The listing builds one solid part. Answer for the finished solid, in the listing's coordinates (mm). A direction names the side the tool comes from. Coordinates: 2 decimals unless noted, no trailing zeros. Write each loop counter-clockwise with the first axis right and the second up, starting at its lowest first coordinate (ties: lowest second). Pieces come first, ordered by that corner, then holes. Notation, with made-up numbers: M 55,40 L 89,40 A6 cw 89,47 Z; hole C 7,51.5 d2. An arc over 180 degrees is marked long. Answer as CSV lines item,"result".
```python
from build123d import *

# Parameters (mm, degrees)
SKETCH1_W           = 54.8
SKETCH1_H           = 53.53
BOSS_EXTRUDE1_DEPTH = 41.6
SKETCH2_W           = 51.6
SKETCH2_H           = 50.33
CUT_EXTRUDE1_DEPTH  = 39.6
SKETCH3_W           = 5.48
SKETCH3_H           = 5.48
BOSS_EXTRUDE2_DEPTH = 25
SKETCH4_R           = 1.35
CUT_EXTRUDE2_DEPTH  = 10
CUT_EXTRUDE3_REACH  = 43.6
SKETCH5_R           = 3.5
CUT_EXTRUDE4_REACH  = 43.6
SKETCH6_R           = 3.1
CUT_EXTRUDE5_REACH  = 43.6
SKETCH7_R           = 3.6
CUT_EXTRUDE6_REACH  = 56.8
SKETCH8_R           = 1.25
CUT_EXTRUDE7_REACH  = 56.8
SKETCH10_R          = 1.25
CUT_EXTRUDE8_REACH  = 55.53
SKETCH12_R          = 7.680495542
CUT_EXTRUDE9_REACH  = 55.53
SKETCH13_W          = 22.581735489
SKETCH13_H          = 15.862362247
CUT_EXTRUDE10_REACH = 56.8
SKETCH14_R          = 1.25


with BuildPart() as part:
    # Sketch1 → Boss-Extrude1 (new body)
    with BuildSketch(Plane(origin=(0, 0, 0), x_dir=(1, 0, 0), z_dir=(0, 1, 0))):
        Rectangle(SKETCH1_W, SKETCH1_H)
    extrude(amount=BOSS_EXTRUDE1_DEPTH)

    # Sketch2 → Cut-Extrude1 (cut)
    with BuildSketch(Plane(origin=(0, 41.6, 0), x_dir=(1, 0, 0), z_dir=(0, 1, 0))):
        Rectangle(SKETCH2_W, SKETCH2_H)
    extrude(amount=-CUT_EXTRUDE1_DEPTH, mode=Mode.SUBTRACT)

    # Sketch3 → Boss-Extrude2 (add)
    with BuildSketch(Plane(origin=(0, 2, 0), x_dir=(1, 0, 0), z_dir=(0, 1, 0))):
        with Locations((-23.06, 22.425)):
            Rectangle(SKETCH3_W, SKETCH3_H)
        with Locations((23.06, 22.425)):
            Rectangle(SKETCH3_W, SKETCH3_H)
        with Locations((23.06, -22.425)):
            Rectangle(SKETCH3_W, SKETCH3_H)
    extrude(amount=BOSS_EXTRUDE2_DEPTH)

    # Sketch4 → Cut-Extrude2 (cut)
    with BuildSketch(Plane(origin=(0, 27, 0), x_dir=(1, 0, 0), z_dir=(0, 1, 0))):
        with Locations((-22.86, 22.225)):
            Circle(SKETCH4_R)
        with Locations((22.86, 22.225)):
            Circle(SKETCH4_R)
        with Locations((22.86, -22.217113742)):
            Circle(SKETCH4_R)
    extrude(amount=-CUT_EXTRUDE2_DEPTH, mode=Mode.SUBTRACT)

    # Sketch5 → Cut-Extrude3 (cut, up to next)
    with BuildSketch(Plane(origin=(0, 0, 0), x_dir=(-1, 0, 0), z_dir=(0, -1, 0)), mode=Mode.PRIVATE) as cut_extrude3_sk1:
        with Locations((-12.762863618, 17.186859774)):
            Circle(SKETCH5_R)
    cut_extrude3_tool1 = extrude(cut_extrude3_sk1.sketch, amount=-CUT_EXTRUDE3_REACH, mode=Mode.PRIVATE) & part.part
    add(cut_extrude3_tool1.solids().sort_by_distance((12.762864, 0, -17.18686))[0], mode=Mode.SUBTRACT)
    # Sketch5 → Cut-Extrude3 (cut, up to next)
    with BuildSketch(Plane(origin=(0, 0, 0), x_dir=(-1, 0, 0), z_dir=(0, -1, 0)), mode=Mode.PRIVATE) as cut_extrude3_sk2:
        with Locations((12.108357792, 17.186859774)):
            Circle(SKETCH5_R)
    cut_extrude3_tool2 = extrude(cut_extrude3_sk2.sketch, amount=-CUT_EXTRUDE3_REACH, mode=Mode.PRIVATE) & part.part
    add(cut_extrude3_tool2.solids().sort_by_distance((-12.108358, 0, -17.18686))[0], mode=Mode.SUBTRACT)

    # Sketch6 → Cut-Extrude4 (cut, up to next)
    with BuildSketch(Plane(origin=(0, 0, 0), x_dir=(-1, 0, 0), z_dir=(0, -1, 0)), mode=Mode.PRIVATE) as cut_extrude4_sk1:
        with Locations((-16.908067186, 1.527180262)):
            Circle(SKETCH6_R)
    cut_extrude4_tool1 = extrude(cut_extrude4_sk1.sketch, amount=-CUT_EXTRUDE4_REACH, mode=Mode.PRIVATE) & part.part
    add(cut_extrude4_tool1.solids().sort_by_distance((16.908067, 0, -1.52718))[0], mode=Mode.SUBTRACT)
    # Sketch6 → Cut-Extrude4 (cut, up to next)
    with BuildSketch(Plane(origin=(0, 0, 0), x_dir=(-1, 0, 0), z_dir=(0, -1, 0)), mode=Mode.PRIVATE) as cut_extrude4_sk2:
        with Locations((-8.726744354, 1.527180262)):
            Circle(SKETCH6_R)
    cut_extrude4_tool2 = extrude(cut_extrude4_sk2.sketch, amount=-CUT_EXTRUDE4_REACH, mode=Mode.PRIVATE) & part.part
    add(cut_extrude4_tool2.solids().sort_by_distance((8.726744, 0, -1.52718))[0], mode=Mode.SUBTRACT)

    # Sketch7 → Cut-Extrude5 (cut, up to next)
    with BuildSketch(Plane(origin=(0, 0, 0), x_dir=(-1, 0, 0), z_dir=(0, -1, 0)), mode=Mode.PRIVATE) as cut_extrude5_sk1:
        with Locations((-12.653779314, -10.035756007)):
            Circle(SKETCH7_R)
    cut_extrude5_tool1 = extrude(cut_extrude5_sk1.sketch, amount=-CUT_EXTRUDE5_REACH, mode=Mode.PRIVATE) & part.part
    add(cut_extrude5_tool1.solids().sort_by_distance((12.653779, 0, 10.035756))[0], mode=Mode.SUBTRACT)

    # Sketch8 → Cut-Extrude6 (cut, up to next)
    with BuildSketch(Plane(origin=(27.4, 0, 0), x_dir=(0, 0, -1), z_dir=(1, 0, 0)), mode=Mode.PRIVATE) as cut_extrude6_sk1:
        with Locations((-21.585, 36.49)):
            Circle(SKETCH8_R)
    cut_extrude6_tool1 = extrude(cut_extrude6_sk1.sketch, amount=-CUT_EXTRUDE6_REACH, mode=Mode.PRIVATE) & part.part
    add(cut_extrude6_tool1.solids().sort_by_distance((27.4, 36.49, 21.585))[0], mode=Mode.SUBTRACT)

    # Sketch10 → Cut-Extrude7 (cut, up to next)
    with BuildSketch(Plane.ZY.offset(27.4), mode=Mode.PRIVATE) as cut_extrude7_sk1:
        with Locations((-21.585, 36.49)):
            Circle(SKETCH10_R)
    cut_extrude7_tool1 = extrude(cut_extrude7_sk1.sketch, amount=-CUT_EXTRUDE7_REACH, mode=Mode.PRIVATE) & part.part
    add(cut_extrude7_tool1.solids().sort_by_distance((-27.4, 36.49, -21.585))[0], mode=Mode.SUBTRACT)

    # Sketch12 → Cut-Extrude8 (cut, up to next)
    with BuildSketch(Plane(origin=(0, 0, -26.765), x_dir=(-1, 0, 0), z_dir=(0, 0, -1)), mode=Mode.PRIVATE) as cut_extrude8_sk1:
        with Locations((0, 19.850785186)):
            Circle(SKETCH12_R)
    cut_extrude8_tool1 = extrude(cut_extrude8_sk1.sketch, amount=-CUT_EXTRUDE8_REACH, mode=Mode.PRIVATE) & part.part
    add(cut_extrude8_tool1.solids().sort_by_distance((0, 19.850785, -26.765))[0], mode=Mode.SUBTRACT)

    # Sketch13 → Cut-Extrude9 (cut, up to next)
    with BuildSketch(Plane.XY.offset(26.765), mode=Mode.PRIVATE) as cut_extrude9_sk1:
        with Locations((-11.980612505, 10.431181124)):
            Rectangle(SKETCH13_W, SKETCH13_H)
    cut_extrude9_tool1 = extrude(cut_extrude9_sk1.sketch, amount=-CUT_EXTRUDE9_REACH, mode=Mode.PRIVATE) & part.part
    add(cut_extrude9_tool1.solids().sort_by_distance((-11.980613, 10.431181, 26.765))[0], mode=Mode.SUBTRACT)

    # Sketch14 → Cut-Extrude10 (cut, up to next)
    with BuildSketch(Plane(origin=(27.4, 0, 0), x_dir=(0, 0, -1), z_dir=(1, 0, 0)), mode=Mode.PRIVATE) as cut_extrude10_sk1:
        with Locations((21.585, 36.49)):
            Circle(SKETCH14_R)
    cut_extrude10_tool1 = extrude(cut_extrude10_sk1.sketch, amount=-CUT_EXTRUDE10_REACH, mode=Mode.PRIVATE) & part.part
    add(cut_extrude10_tool1.solids().sort_by_distance((27.4, 36.49, -21.585))[0], mode=Mode.SUBTRACT)


solid = part.part
```
Q1. Find section A-A (y = 39). Give the vertices of the cut face in (x, z) (3 decimals), and give its area (3 significant figures).
Output:
outline,"M -27.4,-26.765 L 27.4,-26.765 L 27.4,26.765 L -27.4,26.765 Z; hole M -25.8,-25.165 L 25.8,-25.165 L 25.8,25.165 L -25.8,25.165 Z"
area,"336 mm2"
Q2. Find section C-C (z = 11.5). Give the vertices of the cut face in (x, y), and give its area (3 significant figures).
Output:
outline,"M -27.4,0 L 9.37,0 L 9.37,2 L -25.8,2 L -25.8,41.6 L -27.4,41.6 Z; M 15.94,0 L 27.4,0 L 27.4,41.6 L 25.8,41.6 L 25.8,2 L 15.94,2 Z"
area,"223 mm2"
Q3. Straight lines are drawn through the part: line 1 (Z direction, x = 22.86, y = 25.25) (3 decimals); line 2 (X direction, y = 8, z = 24); line 3 (Z direction, x = -20, y = 27.5) (3 decimals). For each, find the intervals that lie inside material, in ascending order.
Output:
line 1,"-26.765 to -23.575, -20.875 to -19.685, 19.685 to 20.867, 23.567 to 26.765"
line 2,"-27.4 to -25.8, 20.32 to 27.4"
line 3,"-26.765 to -25.165, 25.165 to 26.765"
Q4. Flat-ended cylindrical pins translate along their axes: pin 1 Ø4.5 at (x, z) = (23, 22.5) entering from +Y; pin 2 Ø2 at (x, z) = (-22.86, -22.225) entering from +Y; pin 3 Ø3 at (x, y) = (-7.5, 6.5) entering from +Z (3 decimals); pin 4 Ø6 at (x, z) = (-23, -22.5) entering from +Y. Find the tip coordinate at first contact, or state that the pin passes through.
Output:
pin 1,"y = 27"
pin 2,"y = 17"
pin 3,"z = -25.165"
pin 4,"y = 41.6"
Q5. Find section B-B (x = 15). Give the vertices of the cut face in (y, z) (3 decimals).
Output:
outline,"M 0,-26.765 L 41.6,-26.765 L 41.6,-25.165 L 2,-25.165 L 2,-19.879 L 0,-19.879 Z; M 0,-14.495 L 2,-14.495 L 2,-3.97 L 0,-3.97 Z; M 0,0.916 L 2,0.916 L 2,7.305 L 0,7.305 Z; M 0,12.766 L 2,12.766 L 2,25.165 L 41.6,25.165 L 41.6,26.765 L 0,26.765 Z"
Q6. For faces 1 (the cylindrical face through (14.044, 0.986, -0.34)), 2 (the cylindrical face through (22.6, 22.1, -20.9)), 3 (the flat face through (-12, 18.362, 26)), determine the directions among +Z, -Z, +X, -X, +Y, -Y from which every point of the face is accessible in a straight line to the end or side of a thin tool.
Output:
face 1,"+Y, -Y"
face 2,"+Y"
face 3,"+Z"
Q7. The mould has two halves that part along Z. Classify faces 4 (the flat face through (-12, 2.5, 26)), 5 (the cylindrical face through (5.863, 0.986, -0.34)), 6 (the flat face through (0, 21, 26.765)): pulls with the +Z half, pulls with the -Z half, needs draft (parallel to the pull), parting line crosses it, or undercut.
Output:
face 4,"needs draft"
face 5,"undercut"
face 6,"pulls with the +Z half"
Q8. Find section D-D (z = -10.5). Give the vertices of the cut face in (x, y), and give its area (3 significant figures).
Output:
outline,"M -27.4,0 L 27.4,0 L 27.4,41.6 L 25.8,41.6 L 25.8,2 L -25.8,2 L -25.8,41.6 L -27.4,41.6 Z"
area,"236 mm2"
